```python
from build123d import *

# Parameters (mm, degrees)
SKETCH1_R           = 3.3
BOSS_EXTRUDE1_DEPTH = 1.5875


with BuildPart() as part:
    # Sketch1 → Boss-Extrude1 (new body)
    with BuildSketch(Plane.XY):
        with BuildLine():
            Line((-68.878774348, 27.170828826), (-69.084500488, 6.833319702))
            Line((-69.084500488, 6.833319702), (3.290042353, 6.101207661))
            Line((3.290042353, 6.101207661), (3.495768493, 26.438716786))
            Line((3.495768493, 26.438716786), (3.495768493, 97.832907794))
            ThreePointArc((3.495768493, 97.832907794), (-40.545204811, 70.545901145), (-68.878774348, 27.170828826))
        make_face()
        with Locations((-47.368063171, 13.042538508)):
            Circle(SKETCH1_R, mode=Mode.SUBTRACT)
        with Locations((-23.266255505, 12.798764706)):
            Circle(SKETCH1_R, mode=Mode.SUBTRACT)
    extrude(amount=BOSS_EXTRUDE1_DEPTH)


solid = part.part
```
The model under review builds one solid part; all positions refer to its coordinate system, in mm. Round coordinates to 2 decimals unless told otherwise and drop trailing zeros. Loops run counter-clockwise (first coordinate to the right, second up) from the corner with the lowest first, then second, coordinate; pieces in that order, holes last. Notation, with made-up numbers: (89, 47) - (94, 47) arc R7 cw to (94, 56) - close; hole circle Ø5 at (28.5, -25). An arc over 180 degrees is marked (long way). Write each question's results on one line, items separated by ' | '. Start each with the question number.
Q1. Wall thickness on line 1 along X through (y, z) = (11, 0.3); line 2 along Y through (x, z) = (-47, 0.75); line 3 along Y through (x, z) = (-46.5, 0.2): over which ranges is each line inside the solid? List them lowest first. Write a range as [from, to].
Q2. Take a section at A-A on x = -25.5. Give the boundary of the cut face in (y, z).
Q3. Take a section at C-C on y = 74. Give the boundary of the cut face in (x, z), plus the area to 3 significant figures.
Q4. Take a section at D-D on x = -58. Give the boundary of the cut face in (y, z), plus the area to 3 significant figures.
Q5. Draft analysis for pull direction Y (two halves, no side actions). For faces 1 (the flat face through (-25, 42, 1.588)), 2 (the cylindrical face through (-49.987, 11.035, 0.783)), 3 (the cylindrical face through (-40.02, 71.055, 0.783)), state which applies: pulls with the +Y half, pulls with the -Y half, needs draft (parallel to the pull), parting line crosses it, or undercut.
Q6. Take a section at B-B on z = 0.6. Give the boundary of the cut face in (x, y), plus the area to 3 significant figures.
Q7. Insertion check: P1, Ø3, axis at x = -25.5, y = 78.5, coming from the -Z side. The pin has a flat end and moves straight along its axis. Give the tip position at first contact, or say it passes through.
Data:
1) line 1: x = [-69.04, -49.96], [-44.78, -26.03], [-20.5, 3.34] | line 2: y = [6.61, 9.76], [16.32, 63.73] | line 3: y = [6.6, 9.86], [16.23, 64.3]
2) outline: (6.39, 0) - (10.37, 0) - (10.37, 1.59) - (6.39, 1.59) - close; (15.23, 0) - (83, 0) - (83, 1.59) - (15.23, 1.59) - close
3) outline: (-36.85, 0) - (3.5, 0) - (3.5, 1.59) - (-36.85, 1.59) - close | area: 64.1 mm²
4) outline: (6.72, 0) - (49, 0) - (49, 1.59) - (6.72, 1.59) - close | area: 67.1 mm²
5) face 1: needs draft | face 2: undercut | face 3: pulls with the +Y half
6) outline: (-69.08, 6.83) - (3.29, 6.1) - (3.5, 26.44) - (3.5, 97.83) arc R119.38 ccw to (-68.88, 27.17) - close; hole circle Ø6.6 at (-47.37, 13.04); hole circle Ø6.6 at (-23.27, 12.8) | area: 4,750 mm²
7) P1: stops at z = 0
